Job drawing, mm, ordinate dimensions from the low corner. One solid piece. Give positions to 0.01 mm unless a question says otherwise; leave off trailing zeros. Write each loop counter-clockwise with the first axis right and the second up, starting at its lowest first coordinate (ties: lowest second). Pieces come first, ordered by that corner, then holes. Notation, with made-up numbers: M -31.5,15.25 L -17.5,15.25 A30 cw -17.5,44.25 Z; hole C 81,4.5 d3. An arc over 180 degrees is marked long. Use a Markdown table: item, result.
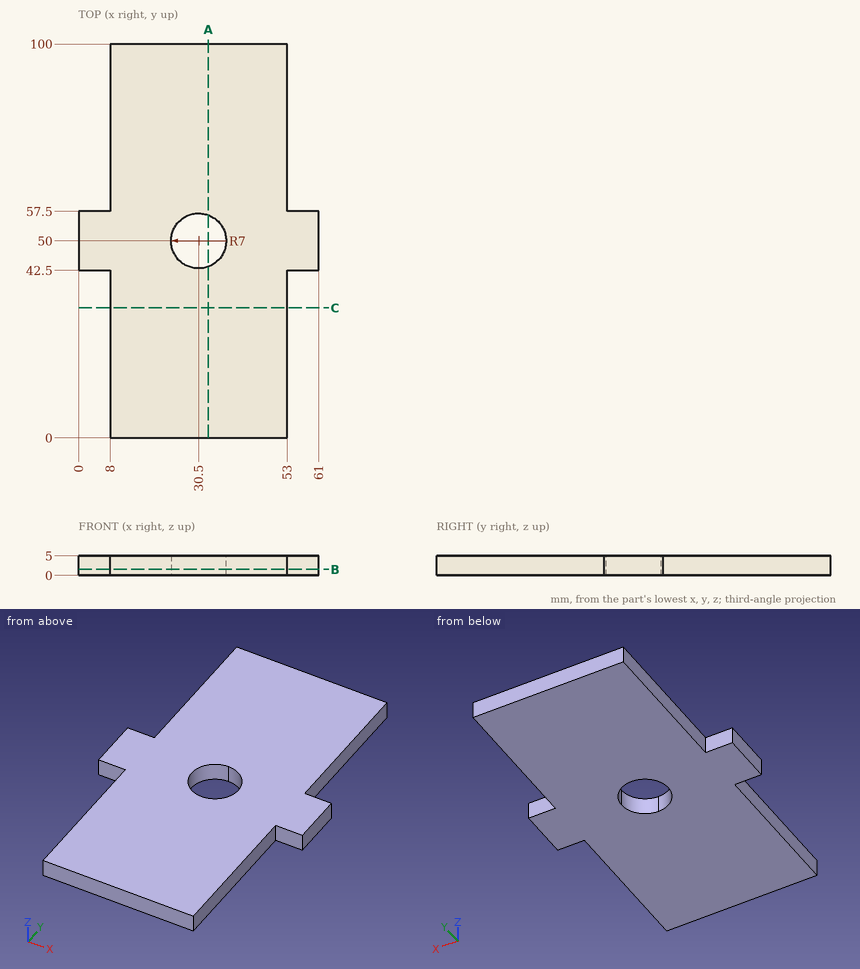
1. Cut at C-C, the plane y = 33. Give the cut face in (x, z).
Findings below:
| item | result |
|---|---|
| outline | M 8,0 L 53,0 L 53,5 L 8,5 Z |
2. Drill centre lines: L1, parallel to X at y = 73.5, z = 0.95; L2, parallel to X at y = 53, z = 0.4; L3, parallel to Y at x = 57.5, z = 1.5. Where is each one in solid material? Low to high.
Findings below:
| item | result |
|---|---|
| L1 | 8 to 53 |
| L2 | 0 to 24.18, 36.82 to 61 |
| L3 | 42.5 to 57.5 |
3. Drop flat-ended pins along their axis: P1, Ø1.5, axis at y = 19.5, z = 4, coming from the -X side; P2, Ø2.5, axis at x = 2.5, z = 3, coming from the -Y side; P3, Ø1.5, axis at y = 22, z = 3.5, coming from the +X side. Give the stop position or say it passes through.
Findings below:
| item | result |
|---|---|
| P1 | x = 8 |
| P2 | y = 42.5 |
| P3 | x = 53 |
4. Cut at A-A, the plane x = 33. Give the cut face in (y, z), then the cut area to 3 significant figures.
Findings below:
| item | result |
|---|---|
| outline | M 0,0 L 43.46,0 L 43.46,5 L 0,5 Z; M 56.54,0 L 100,0 L 100,5 L 56.54,5 Z |
| area | 435 mm2 |
5. Cut at B-B, the plane z = 1.55. Give the cut face in (x, y).
Findings below:
| item | result |
|---|---|
| outline | M 0,42.5 L 8,42.5 L 8,0 L 53,0 L 53,42.5 L 61,42.5 L 61,57.5 L 53,57.5 L 53,100 L 8,100 L 8,57.5 L 0,57.5 Z; hole M 30.5,43 A7 ccw 37.5,50 A7 ccw 30.5,57 A7 ccw Z |
